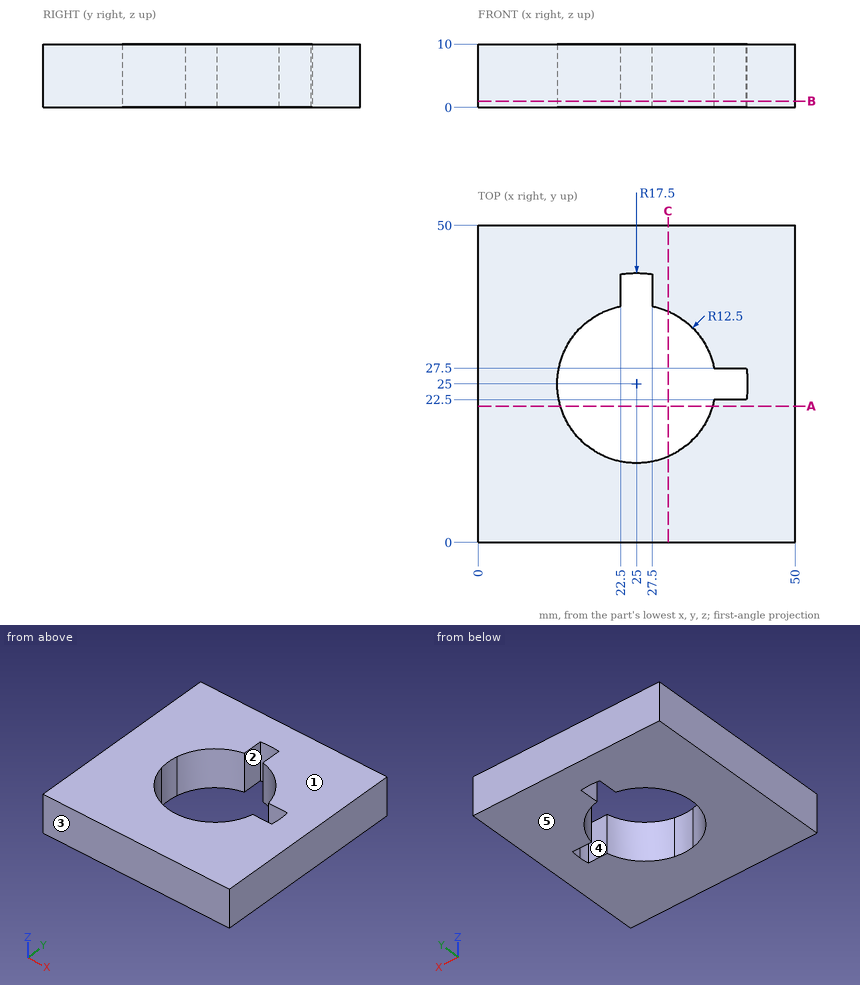
Study the drawing (mm; zero at the part's minimum x, y, z) and answer. A direction names the side the tool comes from. Give positions to 0.01 mm unless a question says otherwise; leave off trailing zeros. Write each loop counter-clockwise with the first axis right and the second up, starting at its lowest first coordinate (ties: lowest second). Pieces come first, ordered by that corner, then holes. Notation, with made-up numbers: (29, 76) - (47, 76) arc R13 ccw to (47, 84) - close; hole circle Ø6 at (75, 23.25). An arc over 180 degrees is marked (long way). One line per question, with ' | ' between items. Start each with the question number.
1. Section A-A, the plane y = 21.5 is taken. Determine the outline of the cut face in (x, z), then the cut area to 3 significant figures.
2. Straight lines are drawn through the part: line 1 (X direction, y = 25.5, z = 8); line 2 (Y direction, x = 40, z = 3.25). For each, find the intervals that lie inside material, in ascending order.
3. Determine the mould class of the marked faces 3, 4 and 5 for opening direction Y: +Y half, -Y half, draft (parallel to the pull), parting line (faces both ways), or undercut.
4. Section B-B, the plane z = 1 is taken. Determine the outline of the cut face in (x, y).
5. For the marked faces 1 and 2, determine the directions among +Z, -Z, +X, -X, +Y, -Y from which every point of the face is accessible in a straight line to the end or side of a thin tool.
6. Section C-C, the plane x = 30 is taken. Determine the outline of the cut face in (y, z), then the cut area to 3 significant figures.
Result:
1) outline: (0, 0) - (13, 0) - (13, 10) - (0, 10) - close; (37, 0) - (50, 0) - (50, 10) - (37, 10) - close | area: 260 mm2
2) line 1: x = 0 to 12.51, 42.49 to 50 | line 2: y = 0 to 22.5, 27.5 to 50
3) face 3: -Y half | face 4: undercut | face 5: draft
4) outline: (0, 0) - (50, 0) - (50, 50) - (0, 50) - close; hole (22.5, 37.25) arc R12.5 ccw (long way) to (37.25, 22.5) - (42.32, 22.5) arc R17.5 ccw to (42.32, 27.5) - (37.25, 27.5) arc R12.5 ccw to (27.5, 37.25) - (27.5, 42.32) arc R17.5 ccw to (22.5, 42.32) - close
5) face 1: +Z, +X, -X, +Y, -Y | face 2: +Z, -Z
6) outline: (0, 0) - (13.54, 0) - (13.54, 10) - (0, 10) - close; (36.46, 0) - (50, 0) - (50, 10) - (36.46, 10) - close | area: 271 mm2
